CAD build for the part. Positions are in the model's coordinates, mm. A direction names the side the tool comes from. Coordinates: 2 decimals unless noted, no trailing zeros. Loops run counter-clockwise (first coordinate to the right, second up) from the corner with the lowest first, then second, coordinate; pieces in that order, holes last. Notation, with made-up numbers: (20.25, 71) -> (33.25, 71) arc R25 cw to (33.25, 89) -> close; hole circle Ø6 at (39.5, 56.5). An arc over 180 degrees is marked (long way). Answer as CSV lines item,"result". Start each with the question number.
from build123d import *

# Parameters (mm, degrees)
BOSS_EXTRUDE1_DEPTH = 3
SKETCH2_R           = 2.3
CUT_EXTRUDE1_DEPTH  = 3


with BuildPart() as part:
    # Sketch1 → Boss-Extrude1 (new body)
    with BuildSketch(Plane.XY):
        Polygon((-20, 12.5), (-20, 10), (-15.2, 10), (-15.2, 12.5), (15.2, 12.5), (15.2, 10), (20, 10), (20, 12.5), (25, 12.5), (25, -12.5), (20, -12.5), (20, -10), (15.2, -10), (15.2, -12.5), (-15.2, -12.5), (-15.2, -10), (-20, -10), (-20, -12.5), (-25, -12.5), (-25, 12.5), align=None)
    extrude(amount=-BOSS_EXTRUDE1_DEPTH)

    # Sketch2 → Cut-Extrude1 (cut)
    with BuildSketch(Plane.XY):
        Circle(SKETCH2_R)
    extrude(amount=-CUT_EXTRUDE1_DEPTH, mode=Mode.SUBTRACT)


solid = part.part
Item 1: Flat gauge pin, fed straight in: pin 1 Ø0.9 at (x, z) = (17, -1.5) entering from -Y. Where does the tip first touch, or does it go through?
Item 2: Saw through at D-D (y = 0). Write the cut outline in (x, z), plus the area to 3 significant figures.
Item 3: Saw through at C-C (x = 0). Write the cut outline in (y, z).
Item 4: Two-plate mould, pull along Y, no slides. Class faces 4 (the face through (0, -12.5, -1)), 5 (the face through (-15.2, 11, -1)), 6 (the face through (-18, 10, -1)), 7 (the face through (-1.825, -1.4, -1.479)): pulls with the +Y half, pulls with the -Y half, needs draft (parallel to the pull), parting line crosses it, or undercut.
Item 5: Wall check: probe 1 along X at (y, z) = (-11, -2.55); probe 2 along Y at (x, z) = (0, -2.05); probe 3 along Y at (x, z) = (17, -0.55). Give the ranges that are in metal, low to high.
Item 6: Saw through at A-A (z = -0.8). Write the cut outline in (x, y), plus the area to 3 significant figures.
Item 7: Saw through at B-B (y = 10.5). Write the cut outline in (x, z), plus the area to 3 significant figures.
Item 8: Which spindle directions (+Z, -Z, +X, -X, +Y, -Y) get a long thin tool onto all of the face, cutting with end or side? Do faces 1 (the face through (15.2, 11, -1)), 2 (the face through (15.2, -11, -1)), 3 (the face through (25, 0, -1)). Say none if no direction does.
Geometry check:
1,pin 1,"y = -10"
2,outline,"(-25, -3) -> (-2.3, -3) -> (-2.3, 0) -> (-25, 0) -> close; (2.3, -3) -> (25, -3) -> (25, 0) -> (2.3, 0) -> close"
2,area,"136 mm2"
3,outline,"(-12.5, -3) -> (-2.3, -3) -> (-2.3, 0) -> (-12.5, 0) -> close; (2.3, -3) -> (12.5, -3) -> (12.5, 0) -> (2.3, 0) -> close"
4,face 4,"pulls with the -Y half"
4,face 5,"needs draft"
4,face 6,"pulls with the +Y half"
4,face 7,"undercut"
5,probe 1,"-25 to -20, -15.2 to 15.2, 20 to 25"
5,probe 2,"-12.5 to -2.3, 2.3 to 12.5"
5,probe 3,"-10 to 10"
6,outline,"(-25, -12.5) -> (-20, -12.5) -> (-20, -10) -> (-15.2, -10) -> (-15.2, -12.5) -> (15.2, -12.5) -> (15.2, -10) -> (20, -10) -> (20, -12.5) -> (25, -12.5) -> (25, 12.5) -> (20, 12.5) -> (20, 10) -> (15.2, 10) -> (15.2, 12.5) -> (-15.2, 12.5) -> (-15.2, 10) -> (-20, 10) -> (-20, 12.5) -> (-25, 12.5) -> close; hole circle Ø4.6 at (0, 0)"
6,area,"1,190 mm2"
7,outline,"(-25, -3) -> (-20, -3) -> (-20, 0) -> (-25, 0) -> close; (-15.2, -3) -> (15.2, -3) -> (15.2, 0) -> (-15.2, 0) -> close; (20, -3) -> (25, -3) -> (25, 0) -> (20, 0) -> close"
7,area,"121 mm2"
8,face 1,"+Z, -Z, +Y"
8,face 2,"+Z, -Z, -Y"
8,face 3,"+Z, -Z, +X, +Y, -Y"
